```python
from build123d import *

# Parameters (mm, degrees)
SKETCH1_R          = 2.725
EXTRUDE1_DEPTH     = 2
CUT_EXTRUDE1_DEPTH = 1
SKETCH3_R          = 1.5
EXTRUDE2_DEPTH     = 10


with BuildPart() as part:
    # Sketch1 → Extrude1 (new body)
    with BuildSketch(Plane.XY):
        Circle(SKETCH1_R)
    extrude(amount=EXTRUDE1_DEPTH)

    # Sketch2 → Cut-Extrude1 (cut)
    with BuildSketch(Plane(origin=(0, 0, 0), x_dir=(-1, 0, 0), z_dir=(0, 0, -1))):
        Polygon((3.449801909, 0), (3.449801909, 0.55), (-3.901269584, 0.55), (-3.901269584, -0.55), (3.449801909, -0.55), align=None)
    extrude(amount=-CUT_EXTRUDE1_DEPTH, mode=Mode.SUBTRACT)

    # Sketch3 → Extrude2 (add)
    with BuildSketch(Plane.XY.offset(2)):
        Circle(SKETCH3_R)
    extrude(amount=EXTRUDE2_DEPTH)


solid = part.part
```
The listing builds one solid part. Answer for the finished solid, in the listing's coordinates (mm). A direction names the side the tool comes from. Round coordinates to 2 decimals unless told otherwise and drop trailing zeros. Write each loop counter-clockwise with the first axis right and the second up, starting at its lowest first coordinate (ties: lowest second). Pieces come first, ordered by that corner, then holes. Notation, with made-up numbers: (8, 5) -> (36, 5) arc R19 ccw to (36, 13) -> close; hole circle Ø2 at (68, -27.5). An arc over 180 degrees is marked (long way). Use CSV: the item, a comma, the result in double quotes. Start each with the question number.
(1) Section D-D on x = -2.4 is taken. Give the vertices of the cut face in (y, z), then the cut area to 3 significant figures.
(2) Section C-C on z = 9.5 is taken. Give the vertices of the cut face in (x, y).
(3) Consider L1, parallel to Z at x = 1.65, y = -1.65; L2, parallel to Y at x = -0.1, z = 11; L3, parallel to Z at x = -1.25, y = -0.25. Determine where each line is inside the solid, lowest interval first. Write a range as from..to.
(4) Section B-B on y = 0 is taken. Give the vertices of the cut face in (x, z) (3 decimals).
(5) Which of the six approach directions +Z, -Z, +X, -X, +Y, -Y give full straight-line access (tool end or side, diameter ignored) to faces 4 (the face through (0, 0, 1)), 5 (the face through (0, 1, 0))?
(6) The mould has two halves that part along Y. Classify faces 1 (the face through (1.2, -1.2, 2)), 2 (the face through (-1.5, 0.07, 6.93)), 3 (the face through (0, 0.55, 0.5)): released by +Y, released by -Y, zero draft, split by the parting line, or undercut.
(7) Section A-A on x = 0 is taken. Give the vertices of the cut face in (y, z) (3 decimals), then the cut area to 3 significant figures.
(8) Each of these flat-tipped pins is pushed along its axis until it touches: pin 1 (0.6 mm diameter, centred on x = 0, y = 0, fed in from -Z); pin 2 (1.5 mm diameter, centred on y = -1.5, z = 6, fed in from +X); pin 3 (1.5 mm diameter, centred on y = 0.5, z = 7, fed in from -X). Where does it stop, or does it pass through?
A:
1,outline,"(-1.29, 0) -> (-0.55, 0) -> (-0.55, 1) -> (0.55, 1) -> (0.55, 0) -> (1.29, 0) -> (1.29, 2) -> (-1.29, 2) -> close"
1,area,"4.06 mm²"
2,outline,"circle Ø3 at (0, 0)"
3,L1,"z = 0..2"
3,L2,"y = -1.5..1.5"
3,L3,"z = 1..12"
4,outline,"(-2.725, 1) -> (2.725, 1) -> (2.725, 2) -> (1.5, 2) -> (1.5, 12) -> (-1.5, 12) -> (-1.5, 2) -> (-2.725, 2) -> close"
5,face 4,"-Z, +X, -X"
5,face 5,"-Z, +X, -X, +Y, -Y"
6,face 1,"zero draft"
6,face 2,"split by the parting line"
6,face 3,"undercut"
7,outline,"(-2.725, 0) -> (-0.55, 0) -> (-0.55, 1) -> (0.55, 1) -> (0.55, 0) -> (2.725, 0) -> (2.725, 2) -> (1.5, 2) -> (1.5, 12) -> (-1.5, 12) -> (-1.5, 2) -> (-2.725, 2) -> close"
7,area,"39.8 mm²"
8,pin 1,"stops at z = 1"
8,pin 2,"stops at x = 1.3"
8,pin 3,"stops at x = -1.5"
